Geometry check sheet. Reference: drawing and pictorial views, mm from the part's lowest x, y, z. A direction names the side the tool comes from. Round coordinates to 2 decimals unless told otherwise and drop trailing zeros. Write each loop counter-clockwise with the first axis right and the second up, starting at its lowest first coordinate (ties: lowest second). Pieces come first, ordered by that corner, then holes. Notation, with made-up numbers: (-13.75, 37) - (31.25, 37) arc R17 cw to (31.25, 43) - close; hole circle Ø8 at (-20.75, 20). An arc over 180 degrees is marked (long way). Use one line per item in the form item = value. Start each with the question number.
1) Set-up check for the marked faces 1 and 2: record each of +Z, -Z, +X, -X, +Y, -Y from which the full face is reachable in a straight line by a thin tool's end or side.
2) Section check C-C (y = 16.5). Record the boundary of the cut face in (x, z).
3) Section check A-A (z = 8). Record the boundary of the cut face in (x, y), then the cut area to 3 significant figures.
4) Section check D-D (x = 14.3). Record the boundary of the cut face in (y, z), then the cut area to 3 significant figures.
5) Gauge pin test, flat ends, axial feed: P1, Ø11, axis at y = 12, z = 20.5, coming from the +X side; P2, Ø10, axis at x = 11, z = 9, coming from the +Y side. Record the tip position at first contact, or that the pin passes through.
6) Section check B-B (x = 2). Record the boundary of the cut face in (y, z).
7) Scan lines: probe 1 along Z at (x, y) = (2.15, 14.3); probe 2 along Y at (x, z) = (8, 23.5). Record each from-to range of solid material in increasing order.
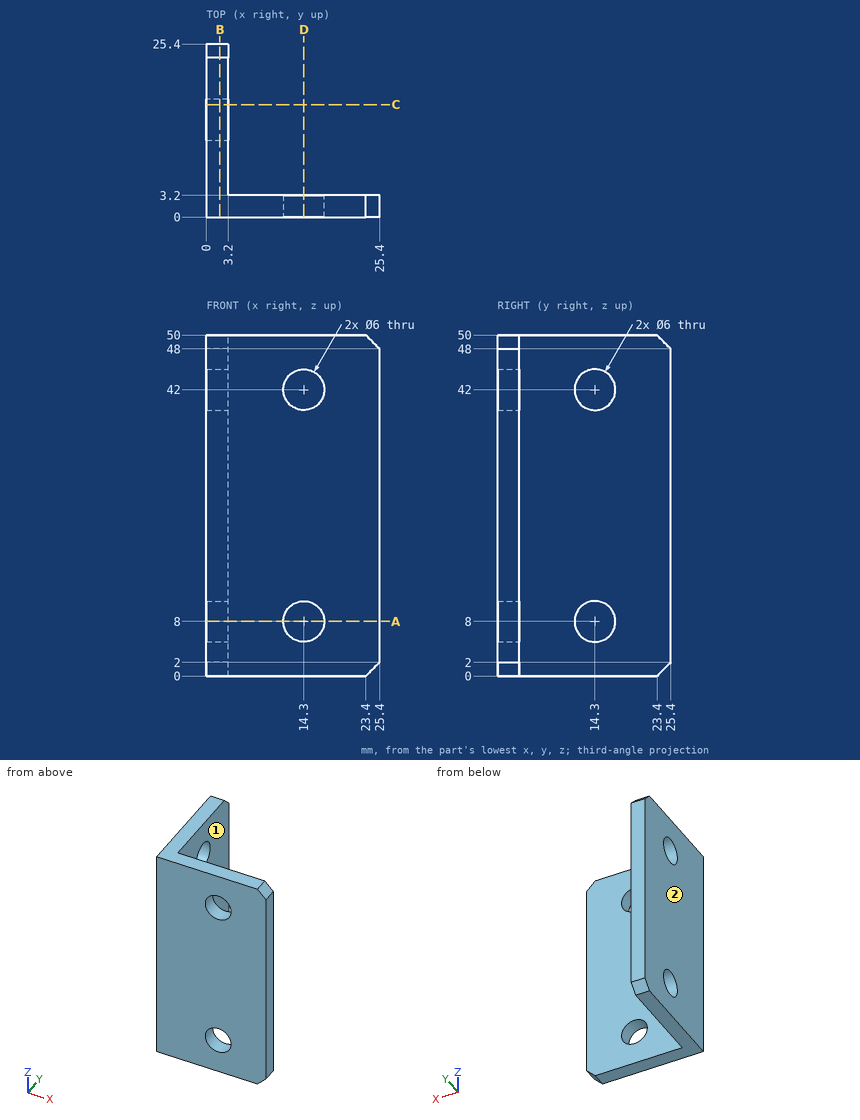
Results are:
q1.face_1 = +Z, -Z, +X, +Y
q1.face_2 = +Z, -Z, -X, +Y, -Y
q2.outline = (0, 0) - (3.2, 0) - (3.2, 5.96) - (0, 5.96) - close; (0, 10.04) - (3.2, 10.04) - (3.2, 39.96) - (0, 39.96) - close; (0, 44.04) - (3.2, 44.04) - (3.2, 50) - (0, 50) - close
q3.outline = (0, 0) - (11.3, 0) - (11.3, 3.2) - (3.2, 3.2) - (3.2, 11.3) - (0, 11.3) - close; (0, 17.3) - (3.2, 17.3) - (3.2, 25.4) - (0, 25.4) - close; (17.3, 0) - (25.4, 0) - (25.4, 3.2) - (17.3, 3.2) - close
q3.area = 114 mm²
q4.outline = (0, 0) - (3.2, 0) - (3.2, 5) - (0, 5) - close; (0, 11) - (3.2, 11) - (3.2, 39) - (0, 39) - close; (0, 45) - (3.2, 45) - (3.2, 50) - (0, 50) - close
q4.area = 122 mm²
q5.P1 = 3.2
q5.P2 = 3.2
q6.outline = (0, 0) - (23.4, 0) - (25.4, 2) - (25.4, 48) - (23.4, 50) - (0, 50) - close; hole circle Ø6 at (14.3, 8); hole circle Ø6 at (14.3, 42)
q7.probe_1 = 0 to 5, 11 to 39, 45 to 50
q7.probe_2 = 0 to 3.2
